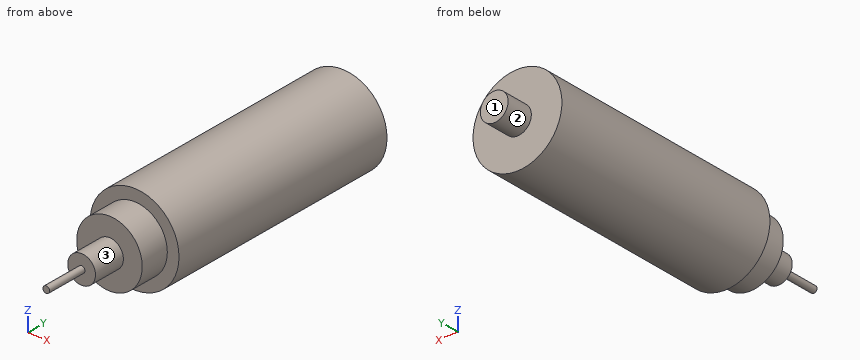
from build123d import *

# Parameters (mm, degrees)
F0_R     = 40
F1_DEPTH = 224
F2_R     = 29.5
F3_DEPTH = 27
F4_R     = 12.5
F5_DEPTH = 30
F6_R     = 12.5
F7_DEPTH = 25
F8_R     = 3
F9_DEPTH = 38


with BuildPart() as f1:
    # F0 (on Front) → F1 (new body)
    with BuildSketch(Plane.XZ):
        Circle(F0_R)
    extrude(amount=F1_DEPTH)

    # F2 (on face) → F3 (join)
    with BuildSketch(Plane.XZ.offset(224)):
        Circle(F2_R)
    extrude(amount=F3_DEPTH)

    # F4 (on face) → F5 (join)
    with BuildSketch(Plane.XZ.offset(251)):
        Circle(F4_R)
    extrude(amount=F5_DEPTH)

    # F6 (on face) → F7 (join)
    with BuildSketch(Plane(origin=(0, 0, 0), x_dir=(-1, 0, 0), z_dir=(0, 1, 0))):
        Circle(F6_R)
    extrude(amount=F7_DEPTH)

    # F8 (on face) → F9 (join)
    with BuildSketch(Plane.XZ.offset(281)):
        Circle(F8_R)
    extrude(amount=F9_DEPTH)


solid = f1.part
Geometry check sheet. Reference: the model listing, model coordinates, mm. Face numbers are marked on the shaded views. A direction names the side the tool comes from. Coordinates: 2 decimals unless noted, no trailing zeros. Loops run counter-clockwise (first coordinate to the right, second up) from the corner with the lowest first, then second, coordinate; pieces in that order, holes last. Notation, with made-up numbers: (55.25, 53) - (84.25, 53) arc R27 ccw to (84.25, 91) - close; hole circle Ø1 at (15, 43). An arc over 180 degrees is marked (long way). Use one line per item in the form item = value. Start each with the question number.
Item 1: Tool access check on the marked faces 1, 2 and 3. Record the directions out of +Z, -Z, +X, -X, +Y, -Y that give a thin tool (end or side, any length) a straight path to the whole face; none if there is none.
Item 2: Section check B-B, the plane x = 0. Enter the section's corners in (y, z).
Item 3: Section check D-D, the plane x = 22. Enter the section's corners in (y, z).
Item 4: Section check C-C, the plane y = -181.5. Enter the section's corners in (x, z).
Item 5: Gauge pin test, flat ends, axial feed: pin 1 (3 mm diameter, centred on x = 13.5, y = -223.5, fed in from -Z); pin 2 (8 mm diameter, centred on x = -5.5, y = -104, fed in from +Z); pin 3 (1.5 mm diameter, centred on x = 24.5, z = 2, fed in from -Y). Record the tip position at first contact, or that the pin passes through.
Item 6: Section check A-A, the plane z = 0. Enter the section's corners in (x, y).
Item 7: Thickness scan on probe 1 along Y at (x, z) = (27, 21.5); probe 2 along Y at (x, z) = (13, -0.5); probe 3 along Z at (x, y) = (-0.5, 10). Record the ranges inside material, lowest first.
Computed:
q1.face_1 = +Z, -Z, +X, -X, +Y
q1.face_2 = +Y
q1.face_3 = -Y
q2.outline = (-319, -3) - (-281, -3) - (-281, -12.5) - (-251, -12.5) - (-251, -29.5) - (-224, -29.5) - (-224, -40) - (0, -40) - (0, -12.5) - (25, -12.5) - (25, 12.5) - (0, 12.5) - (0, 40) - (-224, 40) - (-224, 29.5) - (-251, 29.5) - (-251, 12.5) - (-281, 12.5) - (-281, 3) - (-319, 3) - close
q3.outline = (-251, -19.65) - (-224, -19.65) - (-224, -33.41) - (0, -33.41) - (0, 33.41) - (-224, 33.41) - (-224, 19.65) - (-251, 19.65) - close
q4.outline = circle Ø80 at (0, 0)
q5.pin_1 = -38.16
q5.pin_2 = 39.97
q5.pin_3 = -251
q6.outline = (-40, -224) - (-29.5, -224) - (-29.5, -251) - (-12.5, -251) - (-12.5, -281) - (-3, -281) - (-3, -319) - (3, -319) - (3, -281) - (12.5, -281) - (12.5, -251) - (29.5, -251) - (29.5, -224) - (40, -224) - (40, 0) - (12.5, 0) - (12.5, 25) - (-12.5, 25) - (-12.5, 0) - (-40, 0) - close
q7.probe_1 = -224 to 0
q7.probe_2 = -251 to 0
q7.probe_3 = -12.49 to 12.49
